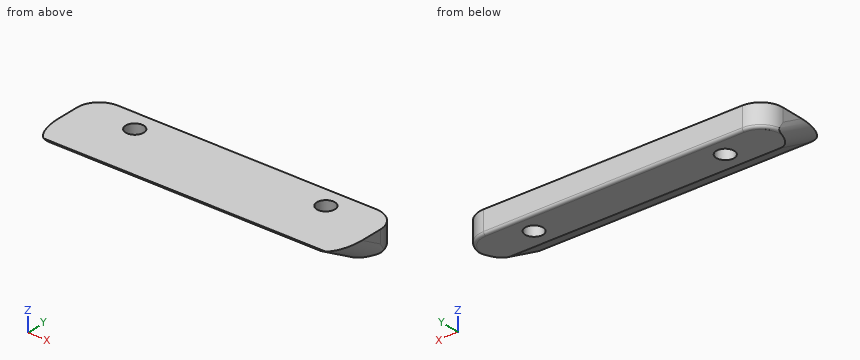
from build123d import *

# Parameters (mm, degrees)
WEDGE_GENERAL_SHAPE_DEPTH       = 73
SKETCH7_W                       = 10
SKETCH7_H                       = 0.2
KNIFE_EDGE_REMOVER_DEPTH        = 74.362115564
FILLET5_R                       = 1.5
FILLET2_START                   = -3
FILLET2_DEPTH                   = 4
BABY_WEDGE_SHORTENER_DEPTH      = 74.362115676
BABY_WEDGE_SHORTENER_DEPTH_BACK = 74.362115676
SKETCH11_W                      = 46
SKETCH11_H                      = 7
FILLET1_R                       = 1.5
FILLET3_START                   = -3
FILLET3_DEPTH                   = 4
BABY_WEDGE_M2_HOLES_D           = 1.6
BITEFILLET_R                    = 0.25


with BuildPart() as part:
    # Sketch2 → Wedge General Shape (new body)
    with BuildSketch(Plane(origin=(0, 0, 0), x_dir=(0, 0, -1), z_dir=(1, 0, 0))):
        Polygon((0, 7), (0, 0), (2, 3.464101615), (2, 7), align=None)
    extrude(amount=WEDGE_GENERAL_SHAPE_DEPTH)

    # Sketch7 → Knife Edge Remover (cut, through all)
    with BuildSketch(Plane(origin=(0, 0, 0), x_dir=(0, 0, -1), z_dir=(1, 0, 0))):
        with Locations((0, 0.1)):
            Rectangle(SKETCH7_W, SKETCH7_H)
    extrude(amount=KNIFE_EDGE_REMOVER_DEPTH, mode=Mode.SUBTRACT)

    # Fillet5
    fillet5_edges = [part.edges().sort_by_distance(p)[0] for p in [
        (73, 1.832050808, -1.057735027),
    ]]
    fillet(fillet5_edges, radius=FILLET5_R)

    # Fillet2: read off the stored shape, not the designer's step
    # Fillet2 outline → Fillet2 (cut)
    with BuildSketch(Plane.XY.offset(FILLET2_START)):
        with BuildLine():
            Line((73, 7), (71, 7))
            ThreePointArc((71, 7), (72.414213562, 6.414213562), (73, 5))
            Line((73, 5), (73, 7))
        make_face()
        with BuildLine():
            ThreePointArc((0, 5), (0.585786438, 6.414213562), (2, 7))
            Line((2, 7), (0, 7))
            Line((0, 7), (0, 5))
        make_face()
    extrude(amount=FILLET2_DEPTH, mode=Mode.SUBTRACT)

    # Sketch11 → Baby Wedge Shortener (cut, two sides: drawn at the far end of the back side and taken through both)
    with BuildSketch(Plane(origin=(0, 0, -2), x_dir=(-1, 0, 0), z_dir=(0, 0, -1)).offset(-BABY_WEDGE_SHORTENER_DEPTH_BACK)):
        with Locations((-23, 3.5)):
            Rectangle(SKETCH11_W, SKETCH11_H)
    extrude(amount=BABY_WEDGE_SHORTENER_DEPTH + BABY_WEDGE_SHORTENER_DEPTH_BACK, mode=Mode.SUBTRACT)

    # Fillet1
    fillet1_edges = [part.edges().sort_by_distance(p)[0] for p in [
        (46, 1.832050808, -1.057735027),
    ]]
    fillet(fillet1_edges, radius=FILLET1_R)

    # Fillet3: read off the stored shape, not the designer's step
    # Fillet3 outline → Fillet3 (cut)
    with BuildSketch(Plane.XY.offset(FILLET3_START)):
        with BuildLine():
            Line((46, 7), (46, 5))
            ThreePointArc((46, 5), (46.585786438, 6.414213562), (48, 7))
            Line((48, 7), (46, 7))
        make_face()
    extrude(amount=FILLET3_DEPTH, mode=Mode.SUBTRACT)

    # Baby Wedge M2 Holes (through all)
    with Locations(Plane(origin=(0, 0, -2), x_dir=(-1, 0, 0), z_dir=(0, 0, -1))):
        with Locations((-68, 5.18), (-51, 5.18)):
            Hole(BABY_WEDGE_M2_HOLES_D / 2)

    # BiteFillet
    bitefillet_edges = [part.edges().sort_by_distance(p)[0] for p in [
        (72.209561466, 6.592784059, -2),
        (46.790438534, 6.592784059, -2),
        (59.5, 7, -2),
    ]]
    fillet(bitefillet_edges, radius=BITEFILLET_R)


solid = part.part
The listing builds one solid part. Answer for the finished solid, in the listing's coordinates (mm). Coordinates: 2 decimals unless noted, no trailing zeros. Write each loop counter-clockwise with the first axis right and the second up, starting at its lowest first coordinate (ties: lowest second). Pieces come first, ordered by that corner, then holes. Notation, with made-up numbers: M -13.5,87 L -3.5,87 A20 ccw -3.5,93 Z; hole C 26.5,70 d6. An arc over 180 degrees is marked long. Write each question's results on one line, items separated by ' | '.
Item 1: The part is cut by section B-B on y = 5.75. State how many separate pieces and enclosed holes the cut face has, and give its area (3 significant figures).
Answer below:
separate pieces: 3 | enclosed holes: 0 | area: 48.9 mm2
Item 2: Given P1, Ø1, axis at x = 57.5, z = -1.5, coming from the -Y side, flat-ended and moving along its own axis, determine where the tip first touches the part or whether it passes through.
Answer below:
P1: y = 1.73
Item 3: Consider probe 1 along X at (y, z) = (5.75, -0.3); probe 2 along X at (y, z) = (4.75, -0.65); probe 3 along Y at (x, z) = (51.5, -0.2). Determine where each line is inside the solid, lowest interval first. Write a range as [from, to].
Answer below:
probe 1: [46.15, 50.44], [51.56, 67.44], [68.56, 72.85] | probe 2: [46, 50.33], [51.67, 67.33], [68.67, 73] | probe 3: [0.35, 4.56], [5.8, 7]
Item 4: The part is cut by section A-A on x = 68. Determine the outline of the cut face in (y, z), and give its area (3 significant figures).
Answer below:
outline: M 0.2,-0.12 L 3.46,-2 L 4.38,-2 L 4.38,0 L 0.2,0 Z; M 5.98,-2 L 6.75,-2 A0.25 ccw 7,-1.75 L 7,0 L 5.98,0 Z | area: 7.31 mm2
